```python
from build123d import *

# Parameters (mm, degrees)
SKETCH1_R           = 22.5
BOSS_EXTRUDE1_DEPTH = 10
BOSS_EXTRUDE2_DEPTH = 20
SKETCH3_R           = 16.5
CUT_EXTRUDE2_DEPTH  = 5


with BuildPart() as part:
    # Sketch1 → Boss-Extrude1 (new body)
    with BuildSketch(Plane(origin=(0, 0, 0), x_dir=(1, 0, 0), z_dir=(0, 1, 0))):
        with Locations(Location((0, 0, 0), (0, 0, 270))):
            Circle(SKETCH1_R)
    extrude(amount=BOSS_EXTRUDE1_DEPTH)

    # Sketch2 → Boss-Extrude2 (add)
    with BuildSketch(Plane(origin=(0, 10, 0), x_dir=(1, 0, 0), z_dir=(0, 1, 0))):
        Polygon((-4.383701715, 27.030528991), (4.446343023, 27.030528991), (25.81653533, -25.886137676), (15.672054161, -25.886137676), (11.559140165, -15.031436821), (-11.47529827, -15.031436821), (-15.598812559, -25.886137676), (-25.743293729, -25.886137676), align=None)
        Polygon((0.036620801, 12.836735588), (-7.871198377, -5.533573573), (7.955040272, -5.533573573), align=None, mode=Mode.SUBTRACT)
    extrude(amount=BOSS_EXTRUDE2_DEPTH)

    # Sketch3 → Cut-Extrude2 (cut)
    with BuildSketch(Plane.XZ):
        with BuildLine():
            ThreePointArc((-14.551420086, 2.778571429), (0, 11.5), (14.551420086, 2.778571429))
            Line((14.551420086, 2.778571429), (4.83856504, 20.948467447))
            ThreePointArc((4.83856504, 20.948467447), (0, 21.5), (-4.83856504, 20.948467447))
            Line((-4.83856504, 20.948467447), (-14.551420086, 2.778571429))
        make_face()
        with Locations((0, -5)):
            Circle(SKETCH3_R)
    extrude(amount=-CUT_EXTRUDE2_DEPTH, mode=Mode.SUBTRACT)


solid = part.part
```
Part model, mm, in its own coordinate system. A direction names the side the tool comes from. Round coordinates to 2 decimals unless told otherwise and drop trailing zeros. Loops run counter-clockwise (first coordinate to the right, second up) from the corner with the lowest first, then second, coordinate; pieces in that order, holes last.
1. Flat gauge pins, fed straight in: pin 1 (10 mm diameter, centred on x = 3.5, y = 15.5, fed in from +Z); pin 2 (2 mm diameter, centred on x = -3, z = 18, fed in from +Y); pin 3 (5 mm diameter, centred on x = -0.5, y = 7.5, fed in from +Z). Where does each tip first touch, or does it go through?
Solutions:
pin 1: stops at z = 15.03
pin 2: stops at y = 10
pin 3: stops at z = 22.5
2. Slice it at D-D (x = -1.5). Give the cut face in (y, z), and give its area (3 significant figures).
Solutions:
outline: (0, -22.45) - (10, -22.45) - (10, -27.03) - (30, -27.03) - (30, -9.27) - (10, -9.27) - (10, 5.53) - (30, 5.53) - (30, 15.03) - (10, 15.03) - (10, 22.45) - (0, 22.45) - (0, 21.45) - (5, 21.45) - (5, -21.43) - (0, -21.43) - close
area: 780 mm2
3. Two-plate mould, pull along X, no slides. Class faces 5 (the face through (15, 19.9, -0.9)), 6 (the face through (4.051, 19.86, -3.523)), 7 (the face through (19, 10, 20)): pulls with the +X half, pulls with the -X half, needs draft (parallel to the pull), parting line crosses it, or undercut.
Solutions:
face 5: pulls with the +X half
face 6: undercut
face 7: needs draft
4. Slice it at A-A (y = 3). Give the cut face in (x, z).
Solutions:
outline: circle Ø45 at (0, 0); hole (-14.55, 2.78) arc R16.5 ccw (long way) to (14.55, 2.78) - (4.84, 20.95) arc R21.5 ccw to (-4.84, 20.95) - close
5. Drill centre lines: line 1 along X through (y, z) = (21.75, 18); line 2 along X through (y, z) = (11.25, -5.5); line 3 along Y through (x, z) = (-14, -7.5). Where is each one in solid material? Low to high.
Solutions:
line 1: x = -22.56 to -12.6, 12.68 to 22.63
line 2: x = -13.07 to -3.12, 3.2 to 13.14
line 3: y = 5 to 10
6. 3-axis set-ups, long thin cutter, end or side, ignore diameter. For faces 1 (the face through (16, 10, -6)), 2 (the face through (-16, 10, -6)), 3 (the face through (-3.86, 19.86, -3.78)), 4 (the face through (-19, 10, 20)): which of +Z, -Z, +X, -X, +Y, -Y reach the whole face in a straight line?
Solutions:
face 1: -Z, +X, +Y
face 2: -Z, -X, +Y
face 3: +Y
face 4: +Z, -X, -Y
7. Slice it at B-B (x = 21). Give the cut face in (y, z), and give its area (3 significant figures).
Solutions:
outline: (0, -8.08) - (10, -8.08) - (10, 8.08) - (0, 8.08) - close; (10, 13.96) - (30, 13.96) - (30, 25.89) - (10, 25.89) - close
area: 400 mm2
8. Slice it at C-C (z = 4.5). Give the cut face in (x, y).
Solutions:
outline: (-22.05, 0) - (-13.63, 0) - (-13.63, 5) - (13.63, 5) - (13.63, 0) - (22.05, 0) - (22.05, 10) - (17.18, 10) - (17.18, 30) - (7.51, 30) - (7.51, 10) - (-7.43, 10) - (-7.43, 30) - (-17.11, 30) - (-17.11, 10) - (-22.05, 10) - close
